```python
from build123d import *

# Parameters (mm, degrees)
SKETCH1_R               = 1.2065
BOSS_EXTRUDE1_DEPTH     = 2.54
SKETCH2_W               = 32.258
SKETCH2_H               = 5.08
BOSS_EXTRUDE2_DEPTH     = 60.96
CUT_EXTRUDE2_DEPTH      = 5.08
SKETCH3_R               = 1.27
CUT_EXTRUDE1_DEPTH      = 5.08
CUT_EXTRUDE3_DEPTH      = 32.258
SKETCH6_R               = 3.21939192
CUT_EXTRUDE4_DEPTH      = 2.54
SKETCH7_R               = 3.216046402
CUT_EXTRUDE5_DEPTH      = 2.54
CUT_EXTRUDE7_DEPTH      = 91.704054458
CUT_EXTRUDE7_DEPTH_BACK = 91.704054458
SKETCH8_W               = 34.637942207
SKETCH8_H               = 68.994690033


with BuildPart() as part:
    # Sketch1 → Boss-Extrude1 (new body)
    with BuildSketch(Plane(origin=(0, 0, 0), x_dir=(1, 0, 0), z_dir=(0, 1, 0))):
        with BuildLine():
            Line((0, 0), (32.258, 0))
            Line((32.258, 0), (32.258, 7.62))
            ThreePointArc((32.258, 7.62), (29.083, 10.795), (25.908, 7.62))
            Line((25.908, 7.62), (6.35, 7.62))
            ThreePointArc((6.35, 7.62), (3.175, 10.795), (0, 7.62))
            Line((0, 7.62), (0, 0))
        make_face()
        with Locations(Location((3.175, 7.62, 0), (0, 0, 270))):
            Circle(SKETCH1_R, mode=Mode.SUBTRACT)
        with Locations(Location((29.083, 7.62, 0), (0, 0, 270))):
            Circle(SKETCH1_R, mode=Mode.SUBTRACT)
    extrude(amount=BOSS_EXTRUDE1_DEPTH)

    # Sketch2 → Boss-Extrude2 (add)
    with BuildSketch(Plane(origin=(0, 2.54, 0), x_dir=(1, 0, 0), z_dir=(0, 1, 0))):
        with Locations((16.129, 2.54)):
            Rectangle(SKETCH2_W, SKETCH2_H)
    extrude(amount=BOSS_EXTRUDE2_DEPTH)

    # Sketch4 → Cut-Extrude2 (cut)
    with BuildSketch(Plane.XY):
        Polygon((32.258, 63.5), (0, 58.42), (0, 63.5), align=None)
    extrude(amount=-CUT_EXTRUDE2_DEPTH, mode=Mode.SUBTRACT)

    # Sketch3 → Cut-Extrude1 (cut)
    with BuildSketch(Plane(origin=(0, 0, -5.08), x_dir=(-1, 0, 0), z_dir=(0, 0, -1))):
        with Locations((-28.767594731, 59.736200914)):
            Circle(SKETCH3_R)
        with Locations((-20.236729821, 58.392757622)):
            Circle(SKETCH3_R)
        with Locations((-11.70586491, 57.049314329)):
            Circle(SKETCH3_R)
        with Locations((-3.175, 55.705871036)):
            Circle(SKETCH3_R)
    extrude(amount=-CUT_EXTRUDE1_DEPTH, mode=Mode.SUBTRACT)

    # Sketch5 → Cut-Extrude3 (cut)
    with BuildSketch(Plane.ZY):
        Polygon((0, 0), (-2.54, 0), (0, 3.81), align=None)
    extrude(amount=-CUT_EXTRUDE3_DEPTH, mode=Mode.SUBTRACT)

    # Sketch6 → Cut-Extrude4 (cut)
    with BuildSketch(Plane(origin=(0.626970779, -3.981264444, 0), x_dir=(0.9878259507117183, 0.1555631418443651, 0), z_dir=(-0.15556314184436507, 0.9878259507117182, 0))):
        with Locations((28.811866038, 7.647867292)):
            Circle(SKETCH6_R)
    extrude(amount=-CUT_EXTRUDE4_DEPTH, mode=Mode.SUBTRACT)

    # Sketch7 → Cut-Extrude5 (cut)
    with BuildSketch(Plane(origin=(0, 0, 0), x_dir=(0.9878259507117183, 0.1555631418443651, 0), z_dir=(-0.15556314184436507, 0.9878259507117182, 0))):
        with Locations((3.216043813, 7.615918666)):
            Circle(SKETCH7_R)
    extrude(amount=-CUT_EXTRUDE5_DEPTH, mode=Mode.SUBTRACT)

    # Mirror1: part across plane


with BuildPart() as part_1:
    add(part.part)
    add(part.part.mirror(Plane(origin=(32.258, 2.54, 0), x_dir=(0, 0, 1), z_dir=(-1, 0, 0))))

    # Sketch8 → Cut-Extrude7 (cut, two sides: drawn at the far end of the back side and taken through both)
    with BuildSketch(Plane(origin=(0, 0, -5.08), x_dir=(-1, 0, 0), z_dir=(0, 0, -1)).offset(-CUT_EXTRUDE7_DEPTH_BACK)):
        with Locations((-14.939028897, 29.002654984)):
            Rectangle(SKETCH8_W, SKETCH8_H)
    extrude(amount=CUT_EXTRUDE7_DEPTH + CUT_EXTRUDE7_DEPTH_BACK, mode=Mode.SUBTRACT)


solid = part_1.part
```
Model file for the job. Use its own axes, mm. A direction names the side the tool comes from. Coordinates: 2 decimals unless noted, no trailing zeros. Loops run counter-clockwise (first coordinate to the right, second up) from the corner with the lowest first, then second, coordinate; pieces in that order, holes last. Notation, with made-up numbers: (79, -12.5) - (114, -12.5) arc R21 cw to (114, 0.5) - close; hole circle Ø4 at (62, 63). An arc over 180 degrees is marked (long way). Write item = value, one per line. Start each with the question number.
Item 1: Wall check: probe 1 along Y at (x, z) = (35.5, -4); probe 2 along Z at (x, y) = (38.5, 37.5); probe 3 along Y at (x, z) = (47.5, -5.25). Give the ranges that are in metal, low to high. Write a range as [from, to].
Item 2: Saw through at A-A, the plane y = 49. List the corners of the cut face in (x, z), then the cut area to 3 significant figures.
Item 3: 3-axis set-ups, long thin cutter, end or side, ignore diameter. For faces 5 (the face through (48, 1, -7.62)), 6 (the face through (49, 2.54, -7)), 7 (the face through (36.61, 1.39, -7.88)): which of +Z, -Z, +X, -X, +Y, -Y reach the whole face in a straight line?
Item 4: Pull direction Y, two halves, no side cores. Call faces 1 (the face through (48.613, 1.878, -1.288)), 2 (the face through (43.34, 59.25, -2.58)), 3 (the face through (61.176, 56.965, -2.576)), 4 (the face through (49, 33, -5.08)): +Y half, -Y half, draft (parallel to the pull), parting line (faces both ways), or undercut.
Item 5: Saw through at B-B, the plane x = 42. List the corners of the cut face in (y, z), then the cut area to 3 significant figures.
Item 6: Drop flat-ended pins along their axis: pin 1 Ø6 at (y, z) = (45, -6) entering from +X; pin 2 Ø4 at (x, z) = (61.341, -7.62) entering from -Y; pin 3 Ø1.5 at (x, z) = (43, -5.5) entering from +Y; pin 4 Ø2 at (x, z) = (49, -5) entering from +Y. Give the stop position or say it passes through.
Answers:
q1.probe_1 = [0, 58.49], [60.98, 62.99]
q1.probe_2 = [-5.08, 0]
q1.probe_3 = [0, 2.54]
q2.outline = (32.26, -5.08) - (64.52, -5.08) - (64.52, 0) - (32.26, 0) - close
q2.area = 164 mm2
q3.face_5 = -Z, +Y, -Y
q3.face_6 = -Z, +X, -X, +Y
q3.face_7 = +Y, -Y
q4.face_1 = -Y half
q4.face_2 = undercut
q4.face_3 = undercut
q4.face_4 = draft
q5.outline = (0, -7.62) - (2.54, -7.62) - (2.54, -5.08) - (61.97, -5.08) - (61.97, 0) - (3.81, 0) - (0, -2.54) - close
q5.area = 316 mm2
q6.pin_1 = 64.52
q6.pin_2 = 0.19
q6.pin_3 = 61.91
q6.pin_4 = 61.02
